Drawing for the job (mm, zero at the part's lowest x, y, z). Round coordinates to 2 decimals unless told otherwise and drop trailing zeros. Loops run counter-clockwise (first coordinate to the right, second up) from the corner with the lowest first, then second, coordinate; pieces in that order, holes last. Notation, with made-up numbers: (77.5, -24) - (115.5, -24) arc R23 ccw to (115.5, 2) - close; hole circle Ø1 at (75.5, -6). An arc over 180 degrees is marked (long way). Put each result on its own line as item: value.
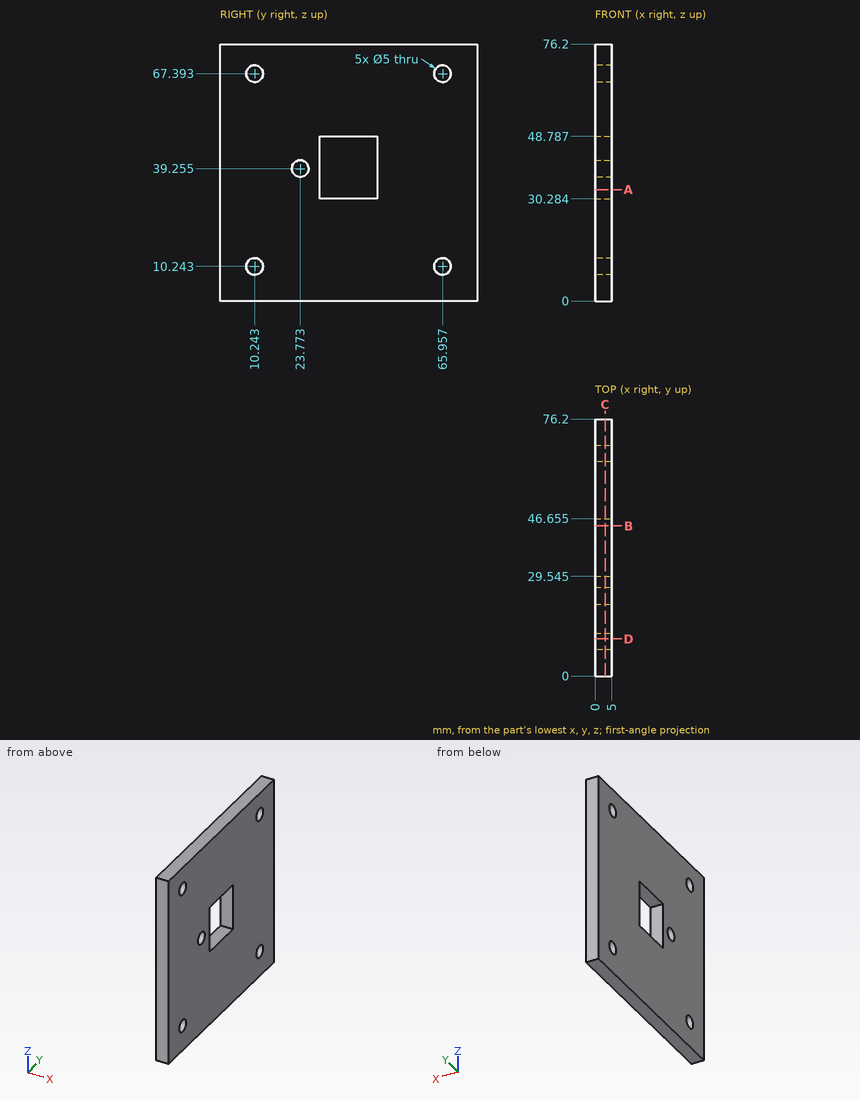
1. Probe line 1 along Y through (x, z) = (2.8, 9.5) (1 decimal); line 2 along Y through (x, z) = (0.75, 46) (1 decimal); line 3 along Z through (x, y) = (1.8, 36). List the from-to ranges inside material, lowest first. Write a range as [from, to].
A:
line 1: y = [0, 7.9], [12.6, 63.6], [68.3, 76.2]
line 2: y = [0, 29.5], [46.7, 76.2]
line 3: z = [0, 30.28], [48.79, 76.2]
2. Band-saw the part on C-C (x = 3). List the corners of the cut face in (y, z) (1 decimal).
A:
outline: (0, 0) - (76.2, 0) - (76.2, 76.2) - (0, 76.2) - close; hole circle Ø5 at (10.2, 10.2); hole circle Ø5 at (10.2, 67.4); hole circle Ø5 at (23.8, 39.3); hole (29.5, 30.3) - (46.7, 30.3) - (46.7, 48.8) - (29.5, 48.8) - close; hole circle Ø5 at (66, 10.2); hole circle Ø5 at (66, 67.4)
3. Band-saw the part on B-B (y = 44.5). List the corners of the cut face in (x, z).
A:
outline: (0, 0) - (5, 0) - (5, 30.28) - (0, 30.28) - close; (0, 48.79) - (5, 48.79) - (5, 76.2) - (0, 76.2) - close
4. Band-saw the part on A-A (z = 33). List the corners of the cut face in (x, y) (1 decimal).
A:
outline: (0, 0) - (5, 0) - (5, 29.5) - (0, 29.5) - close; (0, 46.7) - (5, 46.7) - (5, 76.2) - (0, 76.2) - close
5. Band-saw the part on D-D (y = 11). List the corners of the cut face in (x, z) (1 decimal).
A:
outline: (0, 0) - (5, 0) - (5, 7.9) - (0, 7.9) - close; (0, 12.6) - (5, 12.6) - (5, 65) - (0, 65) - close; (0, 69.8) - (5, 69.8) - (5, 76.2) - (0, 76.2) - close
6. Pin check, flat tip, straight feed: P1, Ø2.5, axis at x = 2.5, z = 37, coming from the -Y side. Stop position of the tip, or through.
A:
P1: stops at y = 0
